Read the model definition and answer for the solid it produces. Units are mm, in the model's axes. A direction names the side the tool comes from. Coordinates: 2 decimals unless noted, no trailing zeros. Write each loop counter-clockwise with the first axis right and the second up, starting at its lowest first coordinate (ties: lowest second). Pieces come first, ordered by that corner, then holes.
1) Each of these flat-tipped pins is pushed along its axis until it touches: pin 1 Ø4 at (x, z) = (-10, 5.5) entering from -Y; pin 2 Ø1 at (x, z) = (-14.5, 9.5) entering from -Y; pin 3 Ø10 at (y, z) = (-72, 12) entering from +X. Where does it stop, or does it pass through?
2) The part is cut by section D-D (y = -76.5). Determine the outline of the cut face in (x, z).
3) Find the intervals of material crossed by line 1 (X direction, y = -29, z = 1); line 2 (Y direction, x = -23, z = 8); line 3 (Y direction, x = -5, z = 3.75), in increasing order.
4) Determine the mould class of faces 1 (the face through (-24, -61, 12)), 2 (the face through (-14.14, -7.605, 4.93)), 3 (the face through (-22.521, -52.127, 14.326)) for opening direction Y: +Y half, -Y half, draft (parallel to the pull), parting line (faces both ways), or undercut.
5) Which of the six approach directions +Z, -Z, +X, -X, +Y, -Y give full straight-line access (tool end or side, diameter ignored) to faces 4 (the face through (-4, -1, 4)), 5 (the face through (-21, -61, 12)), 6 (the face through (-19, -13, 10))?
6) The part is cut by section A-A (z = 11.75). Determine the outline of the cut face in (x, y).
7) The part is cut by section B-B (y = -20.5). Determine the outline of the cut face in (x, z), then the cut area to 3 significant figures.
from build123d import *

# Parameters (mm, degrees)
F1_DEPTH = 10
F3_DEPTH = 3
F4_W     = 3
F4_H     = 60
F5_DEPTH = 10
F6_SIZE  = 9.99999
F8_DEPTH = 25


# Not quite as in the source:
# - a fillet or chamfer is up to 0.001 mm smaller than in the source, because OpenCascade refuses the exact size


with BuildPart() as f1:
    # F0 (on Top) → F1 (new body)
    with BuildSketch(Plane.XY):
        Polygon((20, -15), (0, 0), (0, -3), (17, -15), (17, -90), (20, -90), align=None)
    extrude(amount=F1_DEPTH)

    # F2 (on Front) → F3 (join)
    with BuildSketch(Plane.XZ):
        Polygon((0, 8), (0, 10), (-2, 10), align=None)
    extrude(amount=F3_DEPTH)

    # F4 (on face) → F5 (join)
    with BuildSketch(Plane.XY.offset(10)):
        with Locations((18.5, -60)):
            Rectangle(F4_W, F4_H)
    extrude(amount=F5_DEPTH)

    # F6 (size 10 in the source; OpenCascade refuses exactly that, so slightly less here)
    f6_edges = [f1.edges().sort_by_distance(p)[0] for p in [
        (18.5, -30, 20),
    ]]
    chamfer(f6_edges, length=F6_SIZE)

    # F7 (on face) → F8 (cut)
    with BuildSketch(Plane.YZ.offset(20)):
        with BuildLine():
            Line((-65.3636879024, 0), (-39.5, 0))
            ThreePointArc((-39.5, 0), (-52.4318439512, 14.3294404922), (-65.3636879024, 0))
        make_face()
    extrude(amount=-F8_DEPTH, mode=Mode.SUBTRACT)


with BuildPart() as f10_1:
    # F10: instance of F1
    add(f1.part.mirror(Plane.YZ.offset(-2)))


solid = f10_1.part
Reported:
1. pin 1: stops at y = -8.65
1. pin 2: stops at y = -10.76
1. pin 3: stops at x = -21
2. outline: (-24, 0) - (-21, 0) - (-21, 20) - (-24, 20) - close
3. line 1: x = -24 to -21
3. line 2: y = -90 to -63.59, -41.27 to -14.25
3. line 3: y = -3.71 to -0.75
4. face 1: draft
4. face 2: +Y half
4. face 3: undercut
5. face 4: -Z, +X, +Y, -Y
5. face 5: +Z, -Z, +X, -Y
5. face 6: +Z, +X, -X, +Y
6. outline: (-24, -90) - (-21, -90) - (-21, -60.2) - (-24, -60.2) - close; (-24, -44.66) - (-21, -44.66) - (-21, -31.75) - (-24, -31.75) - close
7. outline: (-24, 0) - (-21, 0) - (-21, 10) - (-24, 10) - close
7. area: 30.0 mm2
